Geometry check sheet. Reference: drawing and pictorial views, mm from the part's lowest x, y, z. Round coordinates to 2 decimals unless told otherwise and drop trailing zeros. Order: outer loops, then holes, each group sorted by start corner. A loop starts at its lowest first (then second) coordinate and runs counter-clockwise, first axis right, second up.
(1) Sectioned sample at A-A, the plane z = 23.5. Count the separate pieces of the cut face and the enclosed holes in it, and give its area (3 significant figures).
(2) Sectioned sample at D-D, the plane x = 13. Enter the section's corners in (y, z), and give its area (3 significant figures).
(3) Depth check by flat-ended pin: pin 1 (9.5 mm diameter, centred on x = 155, y = 18, fed in from +Z); pin 2 (15 mm diameter, centred on x = 120, y = 60, fed in from -Z). Enter the tip coordinate at first touch or a pass-through.
(4) Thickness scan on probe 1 along Y at (x, z) = (15, 26); probe 2 along Y at (x, z) = (122.5, 22.25); probe 3 along Z at (x, y) = (46.5, 22). Record the ranges inside material, lowest first.
(5) Sectioned sample at C-C, the plane x = 155. Enter the section's corners in (y, z).
(6) Sectioned sample at B-B, the plane y = 60. Enter the section's corners in (x, z).
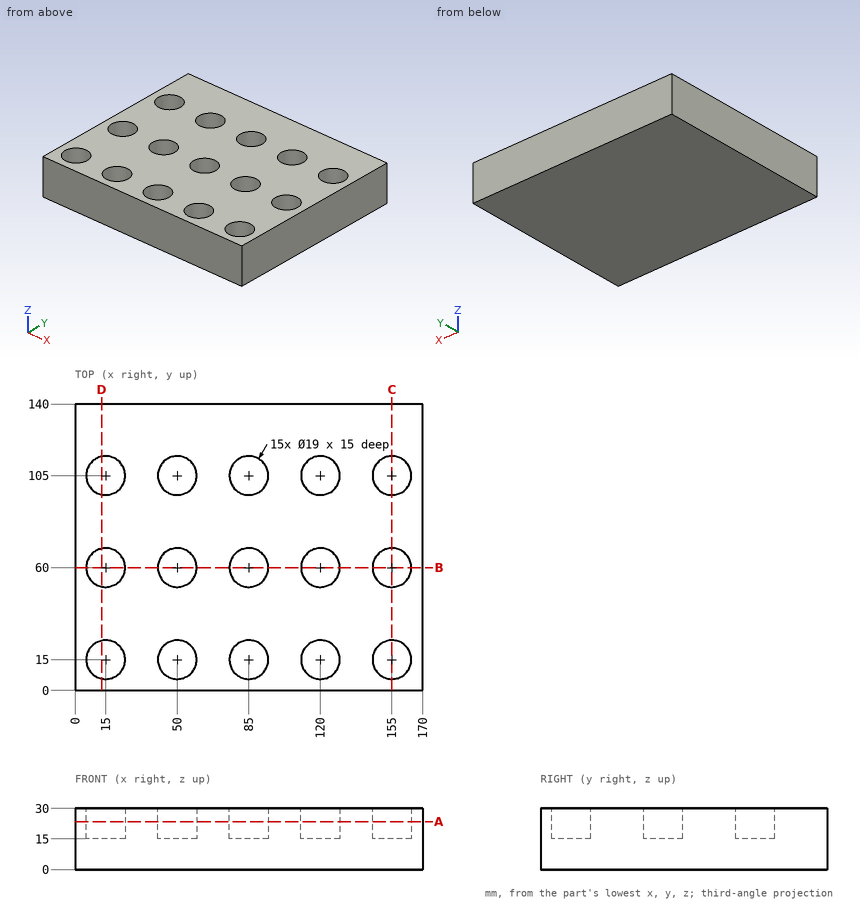
Derived:
1. separate pieces: 1
1. enclosed holes: 15
1. area: 19,500 mm2
2. outline: (0, 0) - (140, 0) - (140, 30) - (114.29, 30) - (114.29, 15) - (95.71, 15) - (95.71, 30) - (69.29, 30) - (69.29, 15) - (50.71, 15) - (50.71, 30) - (24.29, 30) - (24.29, 15) - (5.71, 15) - (5.71, 30) - (0, 30) - close
2. area: 3,360 mm2
3. pin 1: stops at z = 15
3. pin 2: stops at z = 0
4. probe 1: y = 0 to 5.5, 24.5 to 50.5, 69.5 to 95.5, 114.5 to 140
4. probe 2: y = 0 to 5.83, 24.17 to 50.83, 69.17 to 95.83, 114.17 to 140
4. probe 3: z = 0 to 15
5. outline: (0, 0) - (140, 0) - (140, 30) - (114.5, 30) - (114.5, 15) - (95.5, 15) - (95.5, 30) - (69.5, 30) - (69.5, 15) - (50.5, 15) - (50.5, 30) - (24.5, 30) - (24.5, 15) - (5.5, 15) - (5.5, 30) - (0, 30) - close
6. outline: (0, 0) - (170, 0) - (170, 30) - (164.5, 30) - (164.5, 15) - (145.5, 15) - (145.5, 30) - (129.5, 30) - (129.5, 15) - (110.5, 15) - (110.5, 30) - (94.5, 30) - (94.5, 15) - (75.5, 15) - (75.5, 30) - (59.5, 30) - (59.5, 15) - (40.5, 15) - (40.5, 30) - (24.5, 30) - (24.5, 15) - (5.5, 15) - (5.5, 30) - (0, 30) - close
